```python
from build123d import *

# Parameters (mm, degrees)
SKETCH1_W           = 203.2
SKETCH1_H           = 76.2
BOSS_EXTRUDE1_DEPTH = 3.175
SKETCH2_W           = 40.64
SKETCH2_H           = 3.175
CUT_EXTRUDE1_DEPTH  = 3.175
LPATTERN1_COUNT     = 3
LPATTERN1_PITCH     = 81.28
SKETCH3_W           = 3.175
SKETCH3_H           = 15.24
CUT_EXTRUDE2_DEPTH  = 3.175
LPATTERN2_COUNT     = 3
LPATTERN2_PITCH     = 30.48
SKETCH4_R           = 4.7625
SKETCH4_W           = 11.8618
SKETCH4_H           = 11.8618
CUT_EXTRUDE5_DEPTH  = 3.175
SKETCH5_W           = 40.64
SKETCH5_H           = 3.175
CUT_EXTRUDE6_DEPTH  = 3.175


with BuildPart() as part:
    # Sketch1 → Boss-Extrude1 (new body)
    with BuildSketch(Plane(origin=(0, 0, 0), x_dir=(1, 0, 0), z_dir=(0, 1, 0))):
        Rectangle(SKETCH1_W, SKETCH1_H)
    extrude(amount=BOSS_EXTRUDE1_DEPTH)

    # Sketch2 → Cut-Extrude1 (cut)
    with BuildSketch(Plane(origin=(0, 3.175, 0), x_dir=(1, 0, 0), z_dir=(0, 1, 0))):
        with Locations((-81.28, 36.5125)):
            Rectangle(SKETCH2_W, SKETCH2_H)
        with Locations((-81.28, -36.5125)):
            Rectangle(SKETCH2_W, SKETCH2_H)
    cut_extrude1 = extrude(amount=-CUT_EXTRUDE1_DEPTH, mode=Mode.SUBTRACT)

    # LPattern1: Cut-Extrude1 ×3
    with Locations(*[(i * LPATTERN1_PITCH, 0, 0) for i in range(1, LPATTERN1_COUNT)]):
        add(cut_extrude1, mode=Mode.SUBTRACT)

    # Sketch3 → Cut-Extrude2 (cut)
    with BuildSketch(Plane(origin=(0, 3.175, 0), x_dir=(1, 0, 0), z_dir=(0, 1, 0))):
        with Locations((100.0125, 30.48)):
            Rectangle(SKETCH3_W, SKETCH3_H)
        with Locations((-100.0125, 30.48)):
            Rectangle(SKETCH3_W, SKETCH3_H)
    cut_extrude2 = extrude(amount=-CUT_EXTRUDE2_DEPTH, mode=Mode.SUBTRACT)

    # LPattern2: Cut-Extrude2 ×3
    with Locations(*[(0, 0, i * LPATTERN2_PITCH) for i in range(1, LPATTERN2_COUNT)]):
        add(cut_extrude2, mode=Mode.SUBTRACT)

    # Sketch4 → Cut-Extrude5 (cut)
    with BuildSketch(Plane(origin=(0, 3.175, 0), x_dir=(1, 0, 0), z_dir=(0, 1, 0))):
        with Locations((50.8, -18.25625)):
            Circle(SKETCH4_R)
        with Locations((76.099679649, -18.25625)):
            Rectangle(SKETCH4_W, SKETCH4_H)
    extrude(amount=-CUT_EXTRUDE5_DEPTH, mode=Mode.SUBTRACT)

    # Sketch5 → Cut-Extrude6 (cut)
    with BuildSketch(Plane(origin=(0, 3.175, 0), x_dir=(1, 0, 0), z_dir=(0, 1, 0))):
        Rectangle(SKETCH5_W, SKETCH5_H)
    extrude(amount=-CUT_EXTRUDE6_DEPTH, mode=Mode.SUBTRACT)


solid = part.part
```
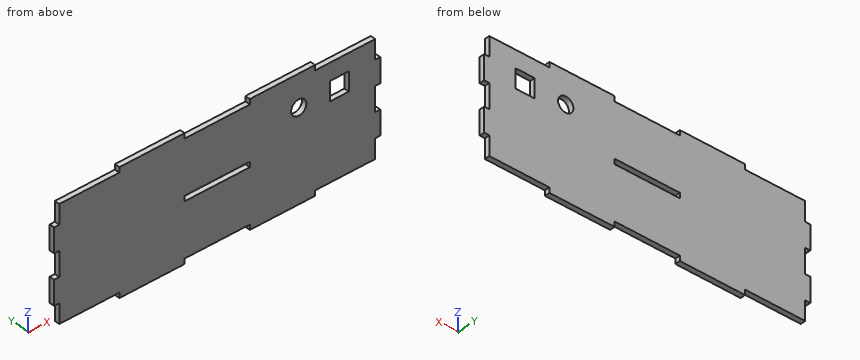
Geometry check sheet. Reference: the model listing, model coordinates, mm. Coordinates: 2 decimals unless noted, no trailing zeros. Order: outer loops, then holes, each group sorted by start corner. A loop starts at its lowest first (then second) coordinate and runs counter-clockwise, first axis right, second up.
Q1. Sectioned sample at B-B on z = -31.5. Record the cut outline in (x, y) (3 decimals).
Reply:
outline: (-98.425, 0) - (98.425, 0) - (98.425, 3.175) - (-98.425, 3.175) - close
Q2. Depth check by flat-ended pin: pin 1 Ø1.6 at (y, z) = (1, 28) entering from +X (3 decimals); pin 2 Ø1.6 at (x, y) = (7, 1) entering from +Z (3 decimals); pin 3 Ø1 at (x, y) = (99.5, 2) entering from -Z. Enter the tip coordinate at first touch or a pass-through.
Reply:
pin 1: stops at x = 98.425
pin 2: stops at z = 34.925
pin 3: stops at z = -22.86
Q3. Sectioned sample at D-D on y = 0.65. Give the number of separate pieces and of enclosed holes in the cut face, and give its area (3 significant figures).
Reply:
separate pieces: 1
enclosed holes: 3
area: 14,100 mm2
Q4. Thickness scan on probe 1 along X at (y, z) = (0.3, 22.5); probe 2 along Z at (x, y) = (78, 1.75) (3 decimals); probe 3 along Z at (x, y) = (50.8, 2.4). Record the ranges inside material, lowest first.
Reply:
probe 1: x = -101.6 to 48.64, 52.96 to 70.17, 82.03 to 101.6
probe 2: z = -34.925 to 12.325, 24.187 to 34.925
probe 3: z = -38.1 to 13.49, 23.02 to 38.1
Q5. Sectioned sample at C-C on x = -63.5. Record the cut outline in (y, z) (3 decimals), and give its area (3 significant figures).
Reply:
outline: (0, -34.925) - (3.175, -34.925) - (3.175, 34.925) - (0, 34.925) - close
area: 222 mm2
Q6. Sectioned sample at A-A on x = 50.8. Record the cut outline in (y, z) (3 decimals).
Reply:
outline: (0, -38.1) - (3.175, -38.1) - (3.175, 13.494) - (0, 13.494) - close; (0, 23.019) - (3.175, 23.019) - (3.175, 38.1) - (0, 38.1) - close
